Geometry: final body of the model. Coordinates: model frame, mm. A direction names the side the tool comes from. Coordinates: 2 decimals unless noted, no trailing zeros. Loops run counter-clockwise (first coordinate to the right, second up) from the corner with the lowest first, then second, coordinate; pieces in that order, holes last. Notation, with made-up numbers: (-10.75, -2.5) - (48.25, -2.5) arc R15 cw to (48.25, 21.5) - close; hole circle Ø9 at (42.25, 47). An arc over 180 degrees is marked (long way). Answer in a Markdown table with one row per item.
Autodesk Inventor part; units mm, degrees
ref_plane "nut_XY" through (6, 0, 0) normal (1, 0, 0) x (0, 0, -1)
ref_plane "nut_YZ" through (6, 0, 0) normal (0, 0, -1) x (0, 1, 0)
ref_plane "nut_ZX" through (6, 0, 0) normal (0, 1, 0) x (1, 0, 0)
sketch "Sketch_1" plane through (0, 0, 0) normal (0, 0, 1) x (1, 0, 0)
  line L0 (6, 0) -> (-4, 0)
  line L1 (-4, 0) -> (-4, 3.1)
  line L2 (-4, 3.1) -> (-3.6, 3.5)
  line L3 (-3.6, 3.5) -> (0, 3.5)
  line L4 (0, 3.5) -> (0, 2)
  line L5 (0, 2) -> (5.5705, 2)
  line L6 (5.5705, 2) -> (6, 1.5705)
  line L7 (6, 1.5705) -> (6, 0)
  line L8 (6, 0) -> (-4, 0)
revolve "Revolution1" add sketch "Sketch_1" angle 360 about axis through (6, 0, 0) along (1, 0, 0)
thread "Thread1"
sketch "Sketch_4" plane through (0, 0, 0) normal (0, 0, 1) x (1, 0, 0)
  line L0 (-1.5981, 0) -> (-4, 0)
  line L1 (-4, 0) -> (-4, 1.5)
  line L2 (-4, 1.5) -> (-2, 1.5)
  line L3 (-2, 1.5) -> (-1.5981, 0)
  line L4 (-1.5981, 0) -> (-4, 0)
revolve "Revolution2" cut sketch "Sketch_4" angle 360 about axis through (-1.5981, 0, 0) along (1, 0, 0)
sketch "Sketch_3" plane through (-4, 0, 0) normal (1, 0, 0) x (0, 0, -1)
  line L0 (-1.5, 0.866) -> (-1.5, -0.866)
  line L1 (-1.5, -0.866) -> (0, -1.7321)
  line L2 (0, -1.7321) -> (1.5, -0.866)
  line L3 (1.5, -0.866) -> (1.5, 0.866)
  line L4 (1.5, 0.866) -> (0, 1.7321)
  line L5 (0, 1.7321) -> (-1.5, 0.866)
extrude "Extrusion1" cut sketch "Sketch_3" along normal blind 2
ref_plane "nut_XY" through (6, 0, 0) normal (1, 0, 0) x (0, 0, -1)
ref_plane "nut_YZ" through (6, 0, 0) normal (0, 0, -1) x (0, 1, 0)
ref_plane "nut_ZX" through (6, 0, 0) normal (0, 1, 0) x (1, 0, 0)
ref_plane "bolt_XY" through (0, 0, 0) normal (1, 0, 0) x (0, 0, -1)
ref_plane "bolt_YZ" through (0, 0, 0) normal (0, 0, -1) x (0, 1, 0)
ref_plane "bolt_ZX" through (0, 0, 0) normal (0, 1, 0) x (1, 0, 0)
properties part number "SCB4-6_1"
(1) Pull-direction query (Z, two-part tool) for faces 1 (the face through (-3.014, 1.293, -0.76)), 2 (the face through (-3.014, 1.305, 0.74)), 3 (the face through (-1.775, 3.233, -1.341)), 4 (the face through (6, 0, 0)); classes: pulls with the +Z half, pulls with the -Z half, needs draft (parallel to the pull), parting line crosses it, or undercut.
Verdict:
| item | result |
|---|---|
| face 1 | undercut |
| face 2 | undercut |
| face 3 | parting line crosses it |
| face 4 | needs draft |
(2) Cut plane A-A on x = 1.25. Output: boundary loops of the cut face in (y, z).
Verdict:
| item | result |
|---|---|
| outline | circle Ø4 at (0, 0) |
(3) First-contact query: pin 1 Ø1 at (x, y) = (2, 1) entering from -Z. Flat tip, straight axial feed; report the tip coordinate or a pass-through.
Verdict:
| item | result |
|---|---|
| pin 1 | stops at z = -1.94 |
(4) Cut plane B-B on x = -1.75. Output: boundary loops of the cut face in (y, z), then the cut area to 3 significant figures.
Verdict:
| item | result |
|---|---|
| outline | circle Ø7 at (0, 0); hole circle Ø1.13 at (0, 0) |
| area | 37.5 mm² |
(5) Access query for faces 5 (the face through (-3, 0, -1.5)), 6 (the face through (-4, 1.3, -1.3)), 7 (the face through (0, 2, -2)). Directions: +Z, -Z, +X, -X, +Y, -Y. A direction counts if a zero-diameter tool reaches every point of the face in a straight line with its end or side. Return the directions, or none.
Verdict:
| item | result |
|---|---|
| face 5 | -X |
| face 6 | +Z, -Z, -X, +Y, -Y |
| face 7 | +X |
(6) Ray query, probe 1 along Y at (x, z) = (4.5, 1); probe 2 along Z at (x, y) = (3.5, 0); probe 3 along X at (y, z) = (-2.5, -0.5). Return the intervals inside material, ascending.
Verdict:
| item | result |
|---|---|
| probe 1 | y = -1.73 to 1.73 |
| probe 2 | z = -2 to 2 |
| probe 3 | x = -4 to 0 |
